Part print with two shaded views. Sizes in mm from the minimum x, y, z corner. A direction names the side the tool comes from. Round coordinates to 2 decimals unless told otherwise and drop trailing zeros. Order: outer loops, then holes, each group sorted by start corner. A loop starts at its lowest first (then second) coordinate and runs counter-clockwise, first axis right, second up. Notation, with made-up numbers: (30.25, -36) -> (56.25, -36) arc R22 ccw to (56.25, -18) -> close; hole circle Ø8 at (76.25, 8.25). An arc over 180 degrees is marked (long way). Answer as a JSON object with one key per item and string values.
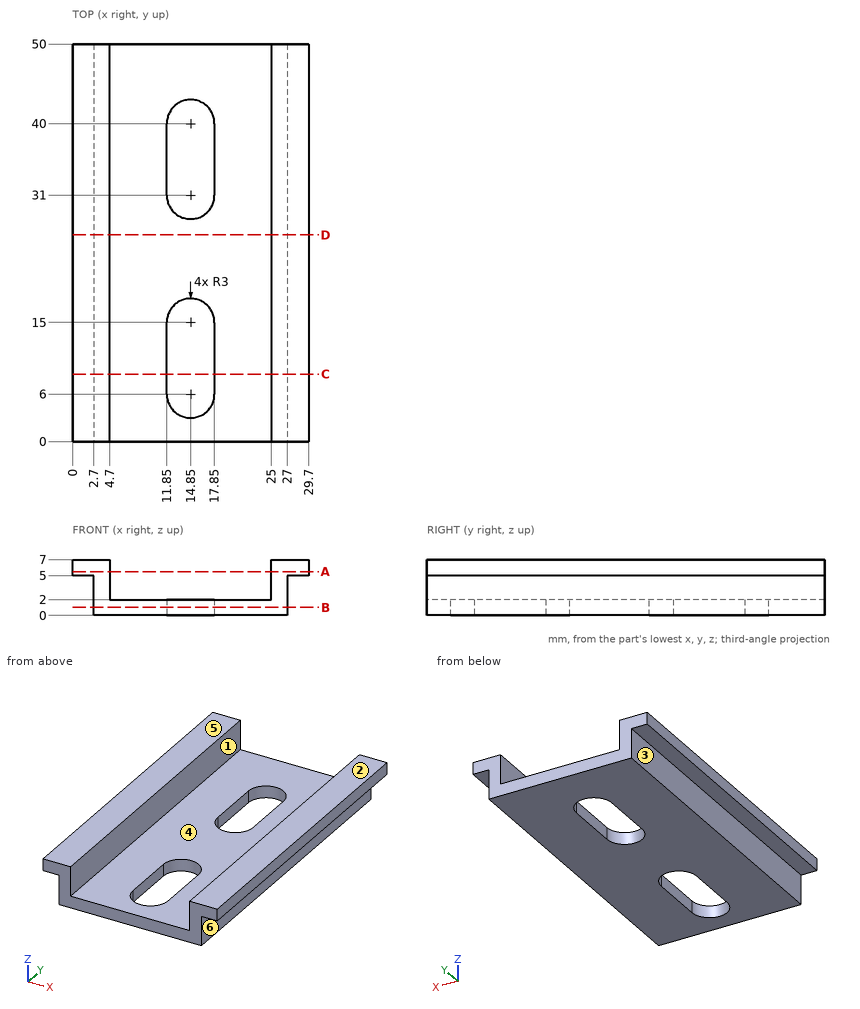
1) Cut at D-D, the plane y = 26. Give the cut face in (x, z), plus the area to 3 significant figures.
Checked values:
{"outline": "(0, 5) -> (2.7, 5) -> (2.7, 0) -> (27, 0) -> (27, 5) -> (29.7, 5) -> (29.7, 7) -> (25, 7) -> (25, 2) -> (4.7, 2) -> (4.7, 7) -> (0, 7) -> close", "area": "79.4 mm²"}
2) Probe L1, parallel to X at y = 44, z = 3; L2, parallel to X at y = 4, z = 5.5; L3, parallel to Z at x = 17, y = 22. List the from-to ranges inside material, lowest first. Write a range as from..to.
Checked values:
{"L1": "x = 2.7..4.7, 25..27", "L2": "x = 0..4.7, 25..29.7", "L3": "z = 0..2"}
3) Pull direction X, two halves, no side cores. Call the marked faces 4, 5 and 6: pulls with the +X half, pulls with the -X half, needs draft (parallel to the pull), parting line crosses it, or undercut.
Checked values:
{"face 4": "undercut", "face 5": "needs draft", "face 6": "pulls with the +X half"}
4) Cut at A-A, the plane z = 5.5. Give the cut face in (x, y).
Checked values:
{"outline": "(0, 0) -> (4.7, 0) -> (4.7, 50) -> (0, 50) -> close; (25, 0) -> (29.7, 0) -> (29.7, 50) -> (25, 50) -> close"}
5) Cut at B-B, the plane z = 1. Give the cut face in (x, y), plus the area to 3 significant figures.
Checked values:
{"outline": "(2.7, 0) -> (27, 0) -> (27, 50) -> (2.7, 50) -> close; hole (11.85, 6) arc R3 ccw to (17.85, 5.97) -> (17.85, 14.97) arc R3 ccw (long way) to (11.85, 15) -> close; hole (11.85, 31) arc R3 ccw to (17.85, 30.97) -> (17.85, 39.97) arc R3 ccw (long way) to (11.85, 40) -> close", "area": "1,050 mm²"}
6) Which spindle directions (+Z, -Z, +X, -X, +Y, -Y) get a long thin tool onto all of the face, cutting with end or side? Do the marked faces 1, 2 and 3. Say none if no direction does.
Checked values:
{"face 1": "+Z, +Y, -Y", "face 2": "+Z, +X, -X, +Y, -Y", "face 3": "-Z, -X, +Y, -Y"}
7) Cut at C-C, the plane y = 8.5. Give the cut face in (x, z).
Checked values:
{"outline": "(0, 5) -> (2.7, 5) -> (2.7, 0) -> (11.85, 0) -> (11.85, 2) -> (4.7, 2) -> (4.7, 7) -> (0, 7) -> close; (17.85, 0) -> (27, 0) -> (27, 5) -> (29.7, 5) -> (29.7, 7) -> (25, 7) -> (25, 2) -> (17.85, 2) -> close"}
8) Flat gauge pins, fed straight in: pin 1 Ø2.5 at (y, z) = (25.5, 3.5) entering from -X; pin 2 Ø6 at (x, y) = (19, 35) entering from -Z; pin 3 Ø1.5 at (x, y) = (7.5, 18) entering from +Z; pin 4 Ø1.6 at (y, z) = (12.5, 1.5) entering from +X. Where does each tip first touch, or does it go through?
Checked values:
{"pin 1": "stops at x = 2.7", "pin 2": "stops at z = 0", "pin 3": "stops at z = 2", "pin 4": "stops at x = 27"}
